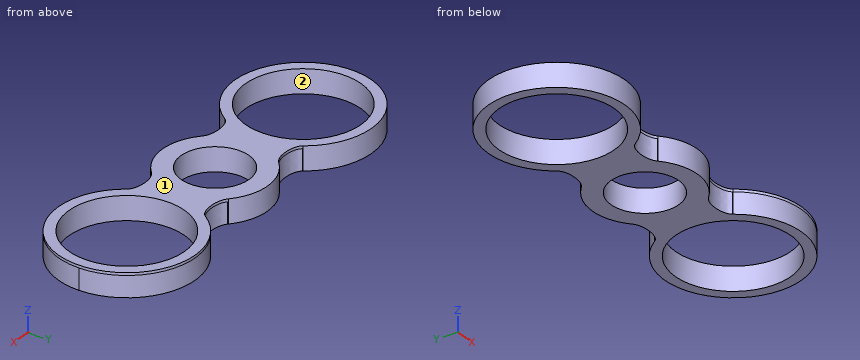
```python
from build123d import *

# Parameters (mm, degrees)
F0_R        = 11.025
F0_R_2      = 8
F0_R_3      = 6.475
F1_DEPTH    = 4
F2_DEPTH    = 4.5
F1_FACE_R   = 11.025
F1_FACE_R_2 = 8
F3_DEPTH    = 0.5


# Not quite as in the source:
# - a feature names something its author has since deleted; it is built from what else it names


with BuildPart() as f1:
    # F0 (on Top) → F1 (new body)
    with BuildSketch(Plane.XY):
        with BuildLine():
            add(Edge.make_bspline(
                [(-13.2970699227, 7.3866190681), (-13.2858031983, 7.3692786835), (-13.2740607617, 7.352142708), (-13.2618542065, 7.3352108101)],
                knots=[0, 0, 0, 0, 0.0117546856, 0.0117546856, 0.0117546856, 0.0117546856], degree=3))
            ThreePointArc((-13.2970699227, 7.3866190681), (-37.05, 0), (-13.2970699227, -7.3866190681))
            add(Edge.make_bspline(
                [(-13.2970699227, -7.3866190681), (-13.2858031983, -7.3692786835), (-13.2740607617, -7.352142708), (-13.2618542065, -7.3352108101)],
                knots=[0, 0, 0, 0, 0.0117546856, 0.0117546856, 0.0117546856, 0.0117546856], degree=3))
            ThreePointArc((-13.2618542065, -7.3352108101), (-11.5783016635, -3.8380106201), (-11, 0))
            ThreePointArc((-11, 0), (-11.5783016635, 3.8380106201), (-13.2618542065, 7.3352108101))
        make_face()
        with Locations((-24.025, 0)):
            Circle(F0_R, mode=Mode.SUBTRACT)
        with BuildLine():
            add(Edge.make_bspline(
                [(13.2970699227, 7.3866190681), (13.2858031983, 7.3692786835), (13.2740607617, 7.352142708), (13.2618542065, 7.3352108101)],
                knots=[0, 0, 0, 0, 0.0117546856, 0.0117546856, 0.0117546856, 0.0117546856], degree=3))
            ThreePointArc((13.2618542065, 7.3352108101), (11, 0), (13.2618542065, -7.3352108101))
            add(Edge.make_bspline(
                [(13.2970699227, -7.3866190681), (13.2858031983, -7.3692786835), (13.2740607617, -7.352142708), (13.2618542065, -7.3352108101)],
                knots=[0, 0, 0, 0, 0.0117546856, 0.0117546856, 0.0117546856, 0.0117546856], degree=3))
            ThreePointArc((13.2970699227, -7.3866190681), (27.8927729861, -12.4374819448), (37.05, 0))
            ThreePointArc((37.05, 0), (27.8927729861, 12.4374819448), (13.2970699227, 7.3866190681))
        make_face()
        with Locations((24.025, 0)):
            Circle(F0_R, mode=Mode.SUBTRACT)
        with BuildLine():
            add(Edge.make_bspline(
                [(-6.9491121946, 7.1909554099), (-6.9214787847, 7.2161071506), (-6.8945995038, 7.2417846871), (-6.8685019311, 7.2679901776)],
                knots=[0.9815772058, 0.9815772058, 0.9815772058, 0.9815772058, 1, 1, 1, 1], degree=3))
            ThreePointArc((-6.9491121946, 7.1909554099), (-10, 0), (-6.9491121946, -7.1909554099))
            add(Edge.make_bspline(
                [(-6.9491121946, -7.1909554099), (-6.9214787847, -7.2161071506), (-6.8945995038, -7.2417846871), (-6.8685019311, -7.2679901776)],
                knots=[0.9815772058, 0.9815772058, 0.9815772058, 0.9815772058, 1, 1, 1, 1], degree=3))
            ThreePointArc((-6.8685019311, -7.2679901776), (0, -10), (6.8685019311, -7.2679901776))
            add(Edge.make_bspline(
                [(6.9491121946, -7.1909554099), (6.9214787847, -7.2161071506), (6.8945995038, -7.2417846871), (6.8685019311, -7.2679901776)],
                knots=[0.9815772058, 0.9815772058, 0.9815772058, 0.9815772058, 1, 1, 1, 1], degree=3))
            ThreePointArc((6.9491121946, -7.1909554099), (9.2057352217, -3.9056931558), (10, 0))
            ThreePointArc((10, 0), (9.2057352217, 3.9056931558), (6.9491121946, 7.1909554099))
            add(Edge.make_bspline(
                [(6.9491121946, 7.1909554099), (6.9214787847, 7.2161071506), (6.8945995038, 7.2417846871), (6.8685019311, 7.2679901776)],
                knots=[0.9815772058, 0.9815772058, 0.9815772058, 0.9815772058, 1, 1, 1, 1], degree=3))
            ThreePointArc((6.8685019311, 7.2679901776), (0, 10), (-6.8685019311, 7.2679901776))
        make_face()
        Circle(F0_R_2, mode=Mode.SUBTRACT)
        Circle(F0_R_2)
        Circle(F0_R_3, mode=Mode.SUBTRACT)
        with BuildLine():
            add(Edge.make_bspline(
                [(-13.2618542065, 7.3352108101), (-12.765654406, 6.6469245328), (-10.2019626219, 5.934402015), (-7.687078337, 6.5192636743), (-6.9491121946, 7.1909554099)],
                knots=[0.0117546856, 0.0117546856, 0.0117546856, 0.0117546856, 0.4895858662, 0.9815772058, 0.9815772058, 0.9815772058, 0.9815772058], degree=3))
            ThreePointArc((-13.2618542065, 7.3352108101), (-11.5783016635, 3.8380106201), (-11, 0))
            ThreePointArc((-11, 0), (-11.5783016635, -3.8380106201), (-13.2618542065, -7.3352108101))
            add(Edge.make_bspline(
                [(-13.2618542065, -7.3352108101), (-12.765654406, -6.6469245328), (-10.2019626219, -5.934402015), (-7.687078337, -6.5192636743), (-6.9491121946, -7.1909554099)],
                knots=[0.0117546856, 0.0117546856, 0.0117546856, 0.0117546856, 0.4895858662, 0.9815772058, 0.9815772058, 0.9815772058, 0.9815772058], degree=3))
            ThreePointArc((-6.9491121946, -7.1909554099), (-10, 0), (-6.9491121946, 7.1909554099))
        make_face()
        with BuildLine():
            add(Edge.make_bspline(
                [(13.2618542065, 7.3352108101), (12.765654406, 6.6469245328), (10.2019626219, 5.934402015), (7.687078337, 6.5192636743), (6.9491121946, 7.1909554099)],
                knots=[0.0117546856, 0.0117546856, 0.0117546856, 0.0117546856, 0.4895858662, 0.9815772058, 0.9815772058, 0.9815772058, 0.9815772058], degree=3))
            ThreePointArc((6.9491121946, 7.1909554099), (9.2057352217, 3.9056931558), (10, 0))
            ThreePointArc((10, 0), (9.2057352217, -3.9056931558), (6.9491121946, -7.1909554099))
            add(Edge.make_bspline(
                [(13.2618542065, -7.3352108101), (12.765654406, -6.6469245328), (10.2019626219, -5.934402015), (7.687078337, -6.5192636743), (6.9491121946, -7.1909554099)],
                knots=[0.0117546856, 0.0117546856, 0.0117546856, 0.0117546856, 0.4895858662, 0.9815772058, 0.9815772058, 0.9815772058, 0.9815772058], degree=3))
            ThreePointArc((13.2618542065, -7.3352108101), (11, 0), (13.2618542065, 7.3352108101))
        make_face()
    extrude(amount=F1_DEPTH)

    # F0 (on Top) → F2 (join)
    with BuildSketch(Plane.XY):
        Circle(F0_R_2)
        Circle(F0_R_3, mode=Mode.SUBTRACT)
    extrude(amount=F2_DEPTH)

    # F1_face (on face) + F0 (on Top) → F3 (join, through all)
    with BuildSketch(Plane.XY.offset(4)):
        with BuildLine():
            ThreePointArc((-6.8685019311, -7.2679901776), (0, -10), (6.8685019311, -7.2679901776))
            add(Edge.make_bspline(
                [(6.8685019311, -7.2679901776), (7.591550229, -6.5419519543), (10.1837329047, -5.9134794065), (12.8278077735, -6.6643873129), (13.2970699227, -7.3866190681)],
                knots=[0.9815772058, 0.9815772058, 0.9815772058, 0.9815772058, 1.4919913396, 1.9815772058, 1.9815772058, 1.9815772058, 1.9815772058], degree=3))
            ThreePointArc((13.2970699227, -7.3866190681), (37.05, 0), (13.2970699227, 7.3866190681))
            add(Edge.make_bspline(
                [(13.2970699227, 7.3866190681), (12.8278077735, 6.6643873129), (10.1837329047, 5.9134794065), (7.591550229, 6.5419519543), (6.8685019311, 7.2679901776)],
                knots=[0, 0, 0, 0, 0.4895858662, 1, 1, 1, 1], degree=3))
            ThreePointArc((6.8685019311, 7.2679901776), (0, 10), (-6.8685019311, 7.2679901776))
            add(Edge.make_bspline(
                [(-6.8685019311, 7.2679901776), (-7.591550229, 6.5419519543), (-10.1837329047, 5.9134794066), (-12.8278077735, 6.6643873129), (-13.2970699227, 7.3866190681)],
                knots=[0.9815772058, 0.9815772058, 0.9815772058, 0.9815772058, 1.4919913396, 1.9815772058, 1.9815772058, 1.9815772058, 1.9815772058], degree=3))
            ThreePointArc((-13.2970699227, 7.3866190681), (-37.05, 0), (-13.2970699227, -7.3866190681))
            add(Edge.make_bspline(
                [(-13.2970699227, -7.3866190681), (-12.8278077735, -6.6643873129), (-10.1837329047, -5.9134794065), (-7.591550229, -6.5419519543), (-6.8685019311, -7.2679901776)],
                knots=[0, 0, 0, 0, 0.4895858662, 1, 1, 1, 1], degree=3))
        make_face()
        with Locations((-24.025, 0)):
            Circle(F1_FACE_R, mode=Mode.SUBTRACT)
        Circle(F1_FACE_R_2, mode=Mode.SUBTRACT)
        with Locations((24.025, 0)):
            Circle(F1_FACE_R, mode=Mode.SUBTRACT)
    with BuildSketch(Plane.XY):
        with BuildLine():
            add(Edge.make_bspline(
                [(-13.2970699227, 7.3866190681), (-13.2858031983, 7.3692786835), (-13.2740607617, 7.352142708), (-13.2618542065, 7.3352108101)],
                knots=[0, 0, 0, 0, 0.0117546856, 0.0117546856, 0.0117546856, 0.0117546856], degree=3))
            ThreePointArc((-13.2970699227, 7.3866190681), (-37.05, 0), (-13.2970699227, -7.3866190681))
            add(Edge.make_bspline(
                [(-13.2970699227, -7.3866190681), (-13.2858031983, -7.3692786835), (-13.2740607617, -7.352142708), (-13.2618542065, -7.3352108101)],
                knots=[0, 0, 0, 0, 0.0117546856, 0.0117546856, 0.0117546856, 0.0117546856], degree=3))
            ThreePointArc((-13.2618542065, -7.3352108101), (-11.5783016635, -3.8380106201), (-11, 0))
            ThreePointArc((-11, 0), (-11.5783016635, 3.8380106201), (-13.2618542065, 7.3352108101))
        make_face()
        with Locations((-24.025, 0)):
            Circle(F0_R, mode=Mode.SUBTRACT)
        with BuildLine():
            add(Edge.make_bspline(
                [(-13.2618542065, 7.3352108101), (-12.765654406, 6.6469245328), (-10.2019626219, 5.934402015), (-7.687078337, 6.5192636743), (-6.9491121946, 7.1909554099)],
                knots=[0.0117546856, 0.0117546856, 0.0117546856, 0.0117546856, 0.4895858662, 0.9815772058, 0.9815772058, 0.9815772058, 0.9815772058], degree=3))
            ThreePointArc((-13.2618542065, 7.3352108101), (-11.5783016635, 3.8380106201), (-11, 0))
            ThreePointArc((-11, 0), (-11.5783016635, -3.8380106201), (-13.2618542065, -7.3352108101))
            add(Edge.make_bspline(
                [(-13.2618542065, -7.3352108101), (-12.765654406, -6.6469245328), (-10.2019626219, -5.934402015), (-7.687078337, -6.5192636743), (-6.9491121946, -7.1909554099)],
                knots=[0.0117546856, 0.0117546856, 0.0117546856, 0.0117546856, 0.4895858662, 0.9815772058, 0.9815772058, 0.9815772058, 0.9815772058], degree=3))
            ThreePointArc((-6.9491121946, -7.1909554099), (-10, 0), (-6.9491121946, 7.1909554099))
        make_face()
        with BuildLine():
            add(Edge.make_bspline(
                [(-6.9491121946, 7.1909554099), (-6.9214787847, 7.2161071506), (-6.8945995038, 7.2417846871), (-6.8685019311, 7.2679901776)],
                knots=[0.9815772058, 0.9815772058, 0.9815772058, 0.9815772058, 1, 1, 1, 1], degree=3))
            ThreePointArc((-6.9491121946, 7.1909554099), (-10, 0), (-6.9491121946, -7.1909554099))
            add(Edge.make_bspline(
                [(-6.9491121946, -7.1909554099), (-6.9214787847, -7.2161071506), (-6.8945995038, -7.2417846871), (-6.8685019311, -7.2679901776)],
                knots=[0.9815772058, 0.9815772058, 0.9815772058, 0.9815772058, 1, 1, 1, 1], degree=3))
            ThreePointArc((-6.8685019311, -7.2679901776), (0, -10), (6.8685019311, -7.2679901776))
            add(Edge.make_bspline(
                [(6.9491121946, -7.1909554099), (6.9214787847, -7.2161071506), (6.8945995038, -7.2417846871), (6.8685019311, -7.2679901776)],
                knots=[0.9815772058, 0.9815772058, 0.9815772058, 0.9815772058, 1, 1, 1, 1], degree=3))
            ThreePointArc((6.9491121946, -7.1909554099), (9.2057352217, -3.9056931558), (10, 0))
            ThreePointArc((10, 0), (9.2057352217, 3.9056931558), (6.9491121946, 7.1909554099))
            add(Edge.make_bspline(
                [(6.9491121946, 7.1909554099), (6.9214787847, 7.2161071506), (6.8945995038, 7.2417846871), (6.8685019311, 7.2679901776)],
                knots=[0.9815772058, 0.9815772058, 0.9815772058, 0.9815772058, 1, 1, 1, 1], degree=3))
            ThreePointArc((6.8685019311, 7.2679901776), (0, 10), (-6.8685019311, 7.2679901776))
        make_face()
        Circle(F0_R_2, mode=Mode.SUBTRACT)
    extrude(amount=F3_DEPTH)


solid = f1.part
```
The listing builds one solid part. Answer for the finished solid, in the listing's coordinates (mm). Face numbers are marked on the shaded views. Give positions to 0.01 mm unless a question says otherwise; leave off trailing zeros. Order: outer loops, then holes, each group sorted by start corner. A loop starts at its lowest first (then second) coordinate and runs counter-clockwise, first axis right, second up. Notation, with made-up numbers: (-33.5, -22) - (-5.5, -22) arc R8 ccw to (-5.5, -15) - close; hole circle Ø1 at (39, 82.25). An arc over 180 degrees is marked (long way). Use one line per item in the form item = value. Start each with the question number.
(1) A cutting plane is placed at A-A, the plane x = 0. Write down the section's boundary in (y, z) (3 decimals).
(2) A cutting plane is placed at C-C, the plane x = -28.5. Write down the section's boundary in (y, z), then the cut area to 3 significant figures.
(3) Flat-ended cylindrical pins translate along their axes: pin 1 Ø11.5 at (x, y) = (0, 0) entering from +Z; pin 2 Ø1.5 at (x, z) = (10, 0.5) entering from +Y; pin 3 Ø2 at (x, z) = (22, 3) entering from +Y; pin 4 Ø1 at (y, z) = (2, 2) entering from +X. Find the tip coordinate at first contact, or state that the pin passes through.
(4) The mould has two halves that part along X. Classify the marked faces 1 and 2: released by +X, released by -X, zero draft, split by the parting line, or undercut.
(5) Consider line 1 (X direction, y = 0.25, z = 1.25); line 2 (Y direction, x = 0, z = 1.15) (3 decimals); line 3 (Y direction, x = 24, z = 4.1). Determine where each line is inside the solid, lowest interval first. Write a range as from..to.
(6) A cutting plane is placed at B-B, the plane z = 0.95. State how many separate pieces and enclosed holes the cut face has, then the cut area to 3 significant figures.
Ans:
q1.outline = (-10, 0) - (-6.475, 0) - (-6.475, 4.5) - (-10, 4.5) - close; (6.475, 0) - (10, 0) - (10, 4.5) - (6.475, 4.5) - close
q2.outline = (-12.23, 0) - (-10.08, 0) - (-10.08, 4.5) - (-12.23, 4.5) - close; (10.08, 0) - (12.23, 0) - (12.23, 4.5) - (10.08, 4.5) - close
q2.area = 19.4 mm^2
q3.pin_1 = through
q3.pin_2 = 6.3
q3.pin_3 = 12.98
q3.pin_4 = 36.96
q4.face_1 = zero draft
q4.face_2 = undercut
q5.line_1 = -37.05..-35.05, -13..-6.47, 6.47..13, 35.05..37.05
q5.line_2 = -10..-6.475, 6.475..10
q5.line_3 = -13.02..-11.02, 11.02..13.02
q6.separate_pieces = 1
q6.enclosed_holes = 3
q6.area = 544 mm^2
